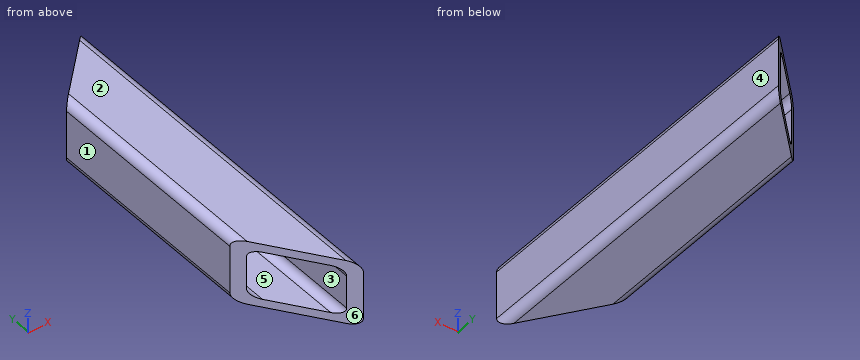
```python
from build123d import *

# Parameters (mm, degrees)
BOSS_EXTRUDE1_DEPTH = 144.78
CUT_EXTRUDE1_DEPTH  = 148.538803032


with BuildPart() as part:
    # Sketch1 → Boss-Extrude1 (new body)
    with BuildSketch(Plane(origin=(0, 0, 0), x_dir=(1, 0, 0), z_dir=(0, 1, 0))):
        with BuildLine():
            Line((-9.398, 0), (9.398, 0))
            ThreePointArc((9.398, 0), (11.732866591, 0.967133409), (12.7, 3.302))
            Line((12.7, 3.302), (12.7, 22.098))
            ThreePointArc((12.7, 22.098), (11.732866591, 24.432866591), (9.398, 25.4))
            Line((9.398, 25.4), (-9.398, 25.4))
            ThreePointArc((-9.398, 25.4), (-11.732866591, 24.432866591), (-12.7, 22.098))
            Line((-12.7, 22.098), (-12.7, 3.302))
            ThreePointArc((-12.7, 3.302), (-11.732866591, 0.967133409), (-9.398, 0))
        make_face()
        with BuildLine():
            Line((-6.477, 3.175), (6.477, 3.175))
            ThreePointArc((6.477, 3.175), (8.632261469, 4.067738531), (9.525, 6.223))
            Line((9.525, 6.223), (9.525, 19.177))
            ThreePointArc((9.525, 19.177), (8.632261469, 21.332261469), (6.477, 22.225))
            Line((6.477, 22.225), (-6.477, 22.225))
            ThreePointArc((-6.477, 22.225), (-8.632261469, 21.332261469), (-9.525, 19.177))
            Line((-9.525, 19.177), (-9.525, 6.223))
            ThreePointArc((-9.525, 6.223), (-8.632261469, 4.067738531), (-6.477, 3.175))
        make_face(mode=Mode.SUBTRACT)
    extrude(amount=BOSS_EXTRUDE1_DEPTH)

    # Sketch2 → Cut-Extrude1 (cut, through all)
    with BuildSketch(Plane.XY):
        Polygon((12.7, 144.78), (-12.7, 119.38), (-12.7, 144.78), align=None)
        Polygon((12.7, 0), (-12.7, 35.56), (-12.7, 0), align=None)
    extrude(amount=-CUT_EXTRUDE1_DEPTH, mode=Mode.SUBTRACT)


solid = part.part
```
The model under review builds one solid part; all positions refer to its coordinate system, in mm. Face numbers are marked on the shaded views. A direction names the side the tool comes from. Coordinates: 2 decimals unless noted, no trailing zeros. Write each loop counter-clockwise with the first axis right and the second up, starting at its lowest first coordinate (ties: lowest second). Pieces come first, ordered by that corner, then holes.
1) To check wall thickness, follow probe 1 along X at (y, z) = (115.5, -15.5) (3 decimals); probe 2 along Z at (x, y) = (1.5, 87) (3 decimals); probe 3 along Z at (x, y) = (-7.25, 114). State the ranges of each line that lie inside material, in increasing order.
2) Machinability: for the marked faces 5 and 6, which of the approach directions +Z, -Z, +X, -X, +Y, -Y give a long, thin tool a straight path to every point of the face, cutting with its end or side? Answer none if there is none.
3) We need section C-C on y = 108.5. State the section outline as (x, z) points (3 decimals).
4) Clearance check with a flat-ended pin moving along its axis: pin 1 Ø1 at (x, z) = (10, -19.5) entering from -Y. State where the tip first meets the part, or that it passes through.
5) We need section B-B on z = -12.5. State the section outline as (x, y) points (3 decimals), then the cut area to 3 significant figures.
6) The part is to be moulded in two halves that separate along X. For the marked faces 1, 2, 3 and 4, say which applies: pulls with the +X half, pulls with the -X half, needs draft (parallel to the pull), parting line crosses it, or undercut.
7) We need section D-D on y = 15.5. State the section outline as (x, z) points (3 decimals).
8) We need section A-A on x = 1.25. State the section outline as (y, z) points (3 decimals).
Answer list:
1. probe 1: x = -12.7 to -9.525, 9.525 to 12.7
1. probe 2: z = -25.4 to -22.225, -3.175 to 0
1. probe 3: z = -25.4 to -22.13, -3.27 to 0
2. face 5: +Y, -Y
2. face 6: +Z, -Z, -X, -Y
3. outline: (-12.7, -22.098) arc R3.302 ccw to (-9.398, -25.4) - (9.398, -25.4) arc R3.302 ccw to (12.7, -22.098) - (12.7, -3.302) arc R3.302 ccw to (9.398, 0) - (-9.398, 0) arc R3.302 ccw to (-12.7, -3.302) - close; hole (-9.525, -19.177) arc R3.048 ccw to (-6.477, -22.225) - (6.477, -22.225) arc R3.048 ccw to (9.525, -19.177) - (9.525, -6.223) arc R3.048 ccw to (6.477, -3.175) - (-6.477, -3.175) arc R3.048 ccw to (-9.525, -6.223) - close
4. pin 1: stops at y = 3.08
5. outline: (-12.7, 35.56) - (-9.525, 31.115) - (-9.525, 122.555) - (-12.7, 119.38) - close; (9.525, 4.445) - (12.7, 0) - (12.7, 144.78) - (9.525, 141.605) - close
5. area: 726 mm2
6. face 1: pulls with the -X half
6. face 2: needs draft
6. face 3: undercut
6. face 4: pulls with the +X half
7. outline: (1.629, -25.4) - (9.398, -25.4) arc R3.302 ccw to (12.7, -22.098) - (12.7, -3.302) arc R3.302 ccw to (9.398, 0) - (1.629, 0) - (1.629, -3.175) - (6.477, -3.175) arc R3.048 cw to (9.525, -6.223) - (9.525, -19.177) arc R3.048 cw to (6.477, -22.225) - (1.629, -22.225) - close
8. outline: (16.03, -25.4) - (133.33, -25.4) - (133.33, -22.225) - (16.03, -22.225) - close; (16.03, -3.175) - (133.33, -3.175) - (133.33, 0) - (16.03, 0) - close
